```python
from build123d import *

# Parameters (mm, degrees)
SKETCH1_W           = 16
SKETCH1_H           = 23
BOSS_EXTRUDE1_DEPTH = 2
SKETCH6_R           = 1.5
BOSS_EXTRUDE3_DEPTH = 1
BOSS_EXTRUDE3_DRAFT = -20


with BuildPart() as part:
    # Sketch1 → Boss-Extrude1 (new body)
    with BuildSketch(Plane.XY):
        with Locations((8, 11.5)):
            Rectangle(SKETCH1_W, SKETCH1_H)
    extrude(amount=BOSS_EXTRUDE1_DEPTH)

    # Loft1: read off the stored shape, not the designer's step
    # Loft1: loft between two sections, ruled curve by curve
    loft1_from = [
        Edge.make_bspline([(10.5, 11.5, 2), (10.5, 16.5, 2), (5.5, 16.5, 2), (5.5, 11.5, 2), (5.5, 6.5, 2), (10.5, 6.5, 2), (10.5, 11.5, 2)], [0, 0, 0, 0, 0.5, 0.5, 0.5, 1, 1, 1, 1], 3, [1, 0.333333333, 0.333333333, 1, 0.333333333, 0.333333333, 1]),
    ]
    loft1_to = [
        Edge.make_bspline([(9.382185261, 10.91727888, 4), (10.547627501, 13.681649403, 4), (7.783256979, 14.847091642, 4), (6.617814739, 12.08272112, 4), (5.452372499, 9.318350597, 4), (8.216743021, 8.152908358, 4), (9.382185261, 10.91727888, 4)], [0, 0, 0, 0, 0.5, 0.5, 0.5, 1, 1, 1, 1], 3, [1, 0.333333333, 0.333333333, 1, 0.333333333, 0.333333333, 1]),
    ]
    loft1 = Solid(Shell([*[Face.make_surface_from_curves(loft1_from[k], loft1_to[k]) for k in range(1)], Face(Wire(loft1_from)), Face(Wire(loft1_to))]))
    add(loft1)


with BuildPart() as boss_extrude3_tool:
    # Sketch6 → Boss-Extrude3 (with draft: the straight prism first)
    with BuildSketch(Plane.XY.offset(4)):
        with Locations((8, 11.5)):
            Circle(SKETCH6_R)
    extrude(amount=BOSS_EXTRUDE3_DEPTH)
    # Boss-Extrude3: the draft: its side faces are tilted about the plane it starts from
    boss_extrude3_sides = [boss_extrude3_tool.faces().sort_by_distance(p)[0] for p in [
        (6.5, 11.5, 4.5),
    ]]
    draft(boss_extrude3_sides, Plane.XY.offset(4), BOSS_EXTRUDE3_DRAFT)


with BuildPart() as part_1:
    add(part.part)

    # Boss-Extrude3: add boss_extrude3_tool
    add(boss_extrude3_tool.part)


solid = part_1.part
```
Can you work these out from the model? Positions are in its coordinate system, mm. Give positions to 0.01 mm unless a question says otherwise; leave off trailing zeros. Loops run counter-clockwise (first coordinate to the right, second up) from the corner with the lowest first, then second, coordinate; pieces in that order, holes last. Notation, with made-up numbers: M 5.5,21.5 L 25.5,21.5 A12 ccw 25.5,28.5 Z; hole C 41.25,-18.75 d7. An arc over 180 degrees is marked long. One line per question, with ' | ' between items. Start each with the question number.
Q1. If we section it at A-A (y = 17.5): Please give me the cut outline in (x, z), plus the area to 3 significant figures.
Q2. If we section it at B-B (x = 3): Please give me the cut outline in (y, z).
Q3. If I drill on line 1 (Z direction, x = 6.25, y = 19.75); line 2 (Y direction, x = 7.25, z = 3.35); line 3 (X direction, y = 10, z = 3.45), over which ranges is the centre line in solid material (lowest first)? Write a range as from..to.
Computed:
1) outline: M 0,0 L 16,0 L 16,2 L 0,2 Z | area: 32.0 mm²
2) outline: M 0,0 L 23,0 L 23,2 L 0,2 Z
3) line 1: z = 0..2 | line 2: y = 9.88..13.12 | line 3: x = 7.12..8.88
